Can you work these out from the model? Positions are in its coordinate system, mm. A direction names the side the tool comes from. Coordinates: 2 decimals unless noted, no trailing zeros. Order: outer loops, then holes, each group sorted by start corner. A loop starts at its lowest first (then second) coordinate and runs counter-clockwise, first axis right, second up. Notation, with made-up numbers: M 25,0.5 L 58,0.5 A25 ccw 58,27.5 Z; hole C 31,-32.75 d8. An arc over 180 degrees is marked long. Answer as CSV lines item,"result". Start each with the question number.
1. If we section it at B-B (z = 1): List the corners of the cut face in (x, y) for me, plus the area to 3 significant figures.
2. On a 3-axis mill with a long thin cutter (end or side, diameter ignored), from which of +Z, -Z, +X, -X, +Y, -Y can I reach the whole of each face in a straight line? I mean faces 1 (the face through (-30, 1, -6)), 2 (the face through (42, 2, 0)), 3 (the face through (30, 1, 6)), 4 (the face through (-42, 2, 0)). Say none if no direction works.
3. Will these pins go through, and if not, where does the flat tip stop? pin 1 (5 mm diameter, centred on x = -19, z = -4.5, fed in from +Y); pin 2 (6 mm diameter, centred on x = 15.5, y = 8, fed in from +Z).
4. I need wall thicknesses on line 1 along Y through (x, z) = (-42, -0.5); line 2 along Z through (x, y) = (23, 13.5); line 3 along X through (y, z) = (3.5, 1.75). Which ranges of each line are inside material? Lowest first, please. Write a range as from..to.
5. If we mould it in two halves opening along X, with no side actions, what happens to faces 5 (the face through (32.66, 10.87, 0.04)), 6 (the face through (-30, 1, 6)), 7 (the face through (-40, 1, 10))? For each: released by +X, released by -X, zero draft, split by the parting line, or undercut.
6. If we section it at D-D (y = 16.75): List the corners of the cut face in (x, z) for me.
7. If we section it at C-C (x = -37.5): List the corners of the cut face in (y, z) for me, plus the area to 3 significant figures.
8. If we section it at A-A (z = -6.5): List the corners of the cut face in (x, y) for me.
```python
from build123d import *

# Parameters (mm, degrees)
PAD_DEPTH    = 2.5
SKETCH001_W  = 20
SKETCH001_H  = 2
PAD001_DEPTH = 10


with BuildPart() as part:
    # Sketch → Pad (new body, symmetric)
    with BuildSketch(Plane.XY):
        Polygon((-50, 0), (50, 0), (50, 2), (40.103793, 2), (25, 20), (-25, 20), (-40.103793, 2), (-50, 2), align=None)
    extrude(amount=PAD_DEPTH, both=True)

    # Sketch001 → Pad001 (join, symmetric)
    with BuildSketch(Plane.XY):
        with Locations((-40, 1)):
            Rectangle(SKETCH001_W, SKETCH001_H)
        with Locations((40, 1)):
            Rectangle(SKETCH001_W, SKETCH001_H)
    extrude(amount=PAD001_DEPTH, both=True)


solid = part.part
```
Solved:
1,outline,"M -50,0 L 50,0 L 50,2 L 40.1,2 L 25,20 L -25,20 L -40.1,2 L -50,2 Z"
1,area,"1,370 mm²"
2,face 1,"-Z, +Y, -Y"
2,face 2,"+X, +Y"
2,face 3,"+Z, +Y, -Y"
2,face 4,"-X, +Y"
3,pin 1,"y = 20"
3,pin 2,"z = 2.5"
4,line 1,"0..2"
4,line 2,"-2.5..2.5"
4,line 3,"-38.85..38.85"
5,face 5,"released by +X"
5,face 6,"undercut"
5,face 7,"zero draft"
6,outline,"M -27.73,-2.5 L 27.73,-2.5 L 27.73,2.5 L -27.73,2.5 Z"
7,outline,"M 0,-10 L 2,-10 L 2,-2.5 L 5.1,-2.5 L 5.1,2.5 L 2,2.5 L 2,10 L 0,10 Z"
7,area,"55.5 mm²"
8,outline,"M -50,0 L -30,0 L -30,2 L -50,2 Z; M 30,0 L 50,0 L 50,2 L 30,2 Z"
